Can you work these out from the model? Positions are in its coordinate system, mm. Face numbers are marked on the shaded views. A direction names the side the tool comes from. Give positions to 0.01 mm unless a question says otherwise; leave off trailing zeros. Order: outer loops, then holes, each group sorted by start corner. A loop starts at its lowest first (then second) coordinate and runs counter-clockwise, first axis right, second up. Notation, with made-up numbers: (67.5, 54) -> (71.5, 54) arc R24 ccw to (71.5, 80) -> close; hole circle Ø1 at (30.5, 10.5). An arc over 180 degrees is marked (long way). Answer as CSV lines item,"result".
```python
from build123d import *

# Parameters (mm, degrees)
SKETCH1_R                  = 38.5
SKETCH1_R_2                = 1.875
SKETCH1_W                  = 36.6
SKETCH1_H                  = 4.6
MAIN_FLANGE_COUPLING_DEPTH = 6
SKETCH2_R                  = 38.5
SKETCH2_R_2                = 1.65
SKETCH2_W                  = 38.8
SKETCH2_H                  = 41.8
BOSS_EXTRUDE1_DEPTH        = 1
SKETCH3_R                  = 3
CUT_EXTRUDE1_DEPTH         = 3


with BuildPart() as part:
    # Sketch1 → Main Flange Coupling (new body)
    with BuildSketch(Plane.XY):
        Circle(SKETCH1_R)
        with Locations((-23.25, 0)):
            Circle(SKETCH1_R_2, mode=Mode.SUBTRACT)
        with Locations((23.25, 0)):
            Circle(SKETCH1_R_2, mode=Mode.SUBTRACT)
        with Locations((0, 4.3)):
            Rectangle(SKETCH1_W, SKETCH1_H, mode=Mode.SUBTRACT)
        with Locations((0, -3.7)):
            Rectangle(SKETCH1_W, SKETCH1_H, mode=Mode.SUBTRACT)
    extrude(amount=-MAIN_FLANGE_COUPLING_DEPTH)

    # Sketch2 → Boss-Extrude1 (add)
    with BuildSketch(Plane.XY):
        with Locations((0.55, -0.25)):
            Circle(SKETCH2_R)
        with Locations((-23.25, 0)):
            Circle(SKETCH2_R_2, mode=Mode.SUBTRACT)
        with Locations((23.25, 0)):
            Circle(SKETCH2_R_2, mode=Mode.SUBTRACT)
        with Locations((0.15, -0.15)):
            Rectangle(SKETCH2_W, SKETCH2_H, mode=Mode.SUBTRACT)
    extrude(amount=BOSS_EXTRUDE1_DEPTH)

    # Sketch3 → Cut-Extrude1 (cut)
    with BuildSketch(Plane.XY.offset(1)):
        with Locations((-23.25, 0)):
            Circle(SKETCH3_R)
        with Locations((23.25, 0)):
            Circle(SKETCH3_R)
    extrude(amount=-CUT_EXTRUDE1_DEPTH, mode=Mode.SUBTRACT)


solid = part.part
```
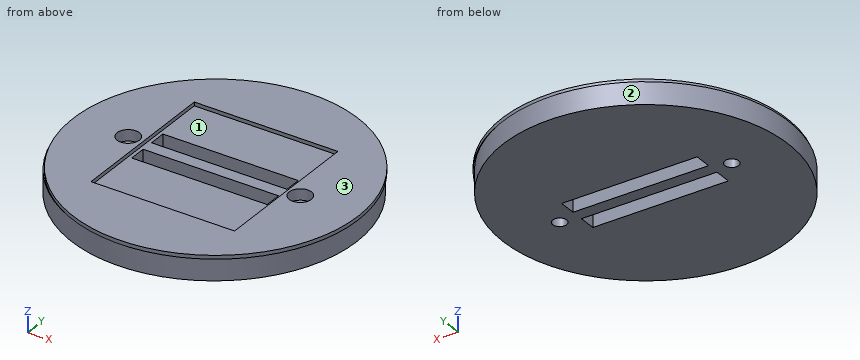
Item 1: For pin 1 (1.4 mm diameter, centred on y = -4, z = -4, fed in from +X); pin 2 (4 mm diameter, centred on x = -14, z = 0, fed in from -Y); pin 3 (3 mm diameter, centred on x = 17, z = -3.5, fed in from +Y); pin 4 (2 mm diameter, centred on x = -30, y = 28.5, fed in from -Z), each with a flat end and sliding along its axis, tell me the tip position at first contact or that it passes through.
Numbers:
pin 1,"stops at x = 38.36"
pin 2,"stops at y = -36.65"
pin 3,"stops at y = 35.24"
pin 4,"passes through"
Item 2: Please list where these lines run through material, in increasing order: line 1 along Y through (x, z) = (-1, -1.75); line 2 along Y through (x, z) = (15.5, -2.5); line 3 along Y through (x, z) = (23.25, -4.9) (3 decimals).
Numbers:
line 1,"y = -38.49 to -6, -1.4 to 2, 6.6 to 38.49"
line 2,"y = -35.24 to -6, -1.4 to 2, 6.6 to 35.24"
line 3,"y = -30.687 to -1.875, 1.875 to 30.687"
Item 3: Imagine slicing it at A-A, the plane z = -3.25. Please give me the cut outline in (x, y) (3 decimals), then the cut area to 3 significant figures.
Numbers:
outline,"circle Ø77 at (0, 0); hole circle Ø3.75 at (-23.25, 0); hole (-18.3, -6) -> (18.3, -6) -> (18.3, -1.4) -> (-18.3, -1.4) -> close; hole (-18.3, 2) -> (18.3, 2) -> (18.3, 6.6) -> (-18.3, 6.6) -> close; hole circle Ø3.75 at (23.25, 0)"
area,"4,300 mm²"
Item 4: Imagine slicing it at D-D, the plane y = 7.5. Please give me the cut outline in (x, z), then the cut area to 3 significant figures.
Numbers:
outline,"(-37.76, -6) -> (37.76, -6) -> (37.76, 0) -> (38.26, 0) -> (38.26, 1) -> (19.55, 1) -> (19.55, 0) -> (-19.25, 0) -> (-19.25, 1) -> (-37.16, 1) -> (-37.16, 0) -> (-37.76, 0) -> close"
area,"490 mm²"
Item 5: For the marked faces 1, 2 and 3, which set-ups out of +Z, -Z, +X, -X, +Y, -Y let a thin tool reach every point of the face, with its end or its side?
Numbers:
face 1,"+Z"
face 2,"-Z"
face 3,"+Z, +X, -X, +Y, -Y"
Item 6: Imagine slicing it at C-C, the plane x = -23.25. Please give me the cut outline in (y, z) (3 decimals).
Numbers:
outline,"(-30.687, -6) -> (-1.875, -6) -> (-1.875, -2) -> (-3, -2) -> (-3, 1) -> (-30.512, 1) -> (-30.512, 0) -> (-30.687, 0) -> close; (1.875, -6) -> (30.687, -6) -> (30.687, 0) -> (30.012, 0) -> (30.012, 1) -> (3, 1) -> (3, -2) -> (1.875, -2) -> close"
Item 7: Imagine slicing it at B-B, the plane x = 0. Please give me the cut outline in (y, z), then the cut area to 3 significant figures.
Numbers:
outline,"(-38.75, 0) -> (-38.5, 0) -> (-38.5, -6) -> (-6, -6) -> (-6, 0) -> (-21.05, 0) -> (-21.05, 1) -> (-38.75, 1) -> close; (-1.4, -6) -> (2, -6) -> (2, 0) -> (-1.4, 0) -> close; (6.6, -6) -> (38.5, -6) -> (38.5, 0) -> (38.25, 0) -> (38.25, 1) -> (20.75, 1) -> (20.75, 0) -> (6.6, 0) -> close"
area,"442 mm²"
